Geometry: see drawing. Coordinates: mm, zero at the bounding-box minimum. A direction names the side the tool comes from. Coordinates: 2 decimals unless noted, no trailing zeros. Loops run counter-clockwise (first coordinate to the right, second up) from the corner with the lowest first, then second, coordinate; pieces in that order, holes last. Notation, with made-up numbers: (53.25, -10.5) - (77.25, -10.5) arc R9 ccw to (77.25, -3.5) - close; hole circle Ø10 at (25.5, 63). An arc over 180 degrees is marked (long way). Use a Markdown table: item, result. Add a question column.
1. Contact query for flat-ended pins moving along their axis: P1, Ø2.5, axis at x = 28, y = 28, coming from the +Z side; P2, Ø2.5, axis at y = 29.5, z = 9, coming from the +X side; P3, Ø0.9, axis at y = 29.5, z = 8, coming from the -X side; P4, Ø0.9, axis at x = 29, z = 9, coming from the +Y side. Output: stop coordinate, or through.
2. Section query C-C on y = 21.5. Return the cut outline in (x, z).
3. Section query A-A on x = 22. Return the cut outline in (y, z).
4. Section query B-B on z = 7.5. Return the cut outline in (x, y), then the cut area to 3 significant figures.
5. Section query D-D on z = 4. State how many separate pieces and enclosed holes the cut face has, then the cut area to 3 significant figures.
6. Ray query, L1, parallel to X at y = 28, z = 5; L2, parallel to X at y = 9.5, z = 7.75; L3, parallel to Y at x = 1.5, z = 4.5. Return the intervals inside material, ascending. Write a range as [from, to].
7. Draft query along X for the marked faces 1, 2 and 3. Return one class per face: released by +X, released by -X, zero draft, split by the parting line, or undercut.
8. Access query for the marked faces 4, 5 and 6. Directions: +Z, -Z, +X, -X, +Y, -Y. A direction counts if a zero-diameter tool reaches every point of the face in a straight line with its end or side. Return the directions, or none.
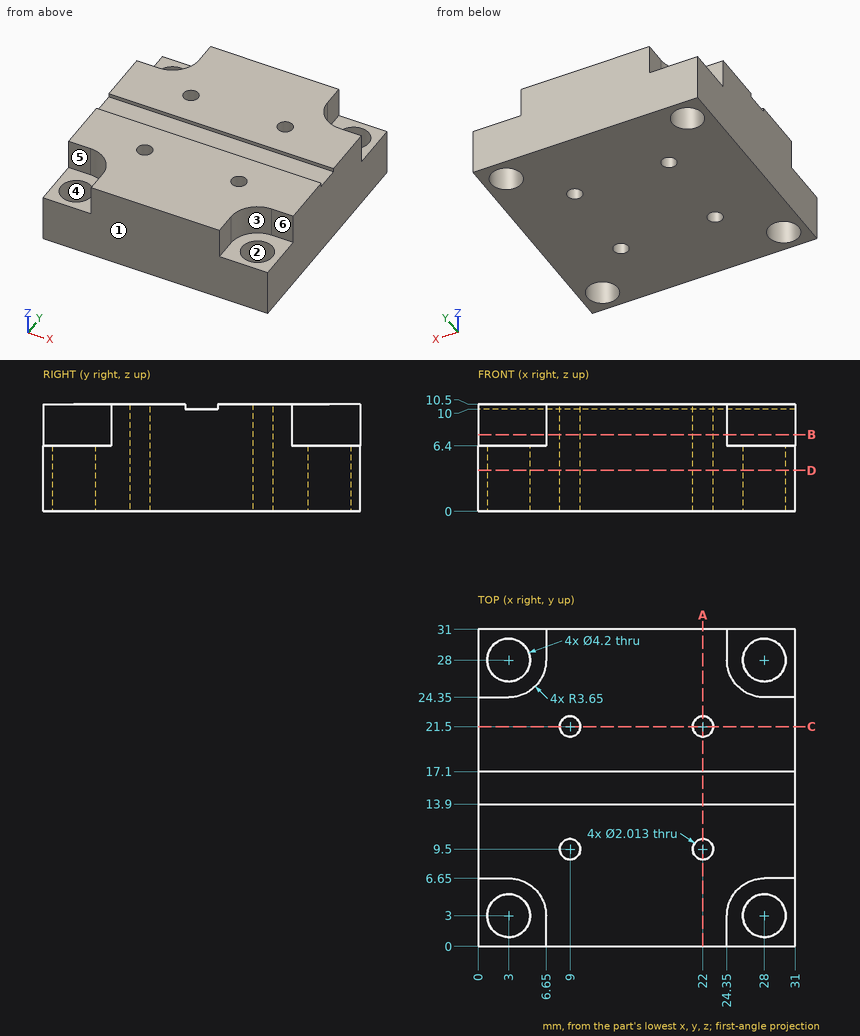
Resolved:
| question | item | result |
|---|---|---|
| 1 | P1 | through |
| 1 | P2 | x = 24.35 |
| 1 | P3 | x = 6.65 |
| 1 | P4 | y = 24.35 |
| 2 | outline | (0, 0) - (7.99, 0) - (7.99, 10.5) - (0, 10.5) - close; (10.01, 0) - (20.99, 0) - (20.99, 10.5) - (10.01, 10.5) - close; (23.01, 0) - (31, 0) - (31, 10.5) - (23.01, 10.5) - close |
| 3 | outline | (0, 0) - (8.49, 0) - (8.49, 10.5) - (0, 10.5) - close; (10.51, 0) - (20.49, 0) - (20.49, 10.5) - (17.1, 10.5) - (17.1, 10) - (13.9, 10) - (13.9, 10.5) - (10.51, 10.5) - close; (22.51, 0) - (31, 0) - (31, 10.5) - (22.51, 10.5) - close |
| 4 | outline | (0, 6.65) - (3, 6.65) arc R3.65 cw to (6.65, 3) - (6.65, 0) - (24.35, 0) - (24.35, 3) arc R3.65 cw to (28, 6.65) - (31, 6.65) - (31, 24.35) - (28, 24.35) arc R3.65 cw to (24.35, 28) - (24.35, 31) - (6.65, 31) - (6.65, 28) arc R3.65 cw to (3, 24.35) - (0, 24.35) - close; hole circle Ø2.01 at (9, 9.5); hole circle Ø2.01 at (9, 21.5); hole circle Ø2.01 at (22, 9.5); hole circle Ø2.01 at (22, 21.5) |
| 4 | area | 783 mm² |
| 5 | separate pieces | 1 |
| 5 | enclosed holes | 8 |
| 5 | area | 893 mm² |
| 6 | L1 | [0, 0.9], [5.1, 25.9], [30.1, 31] |
| 6 | L2 | [0, 7.99], [10.01, 20.99], [23.01, 31] |
| 6 | L3 | [0, 1.53], [4.47, 26.53], [29.47, 31] |
| 7 | face 1 | zero draft |
| 7 | face 2 | undercut |
| 7 | face 3 | released by +X |
| 8 | face 4 | +Z, -Z |
| 8 | face 5 | +Z, -X, -Y |
| 8 | face 6 | +Z, +X, -Y |
